from build123d import *

# Parameters (mm, degrees)
SKETCH_R        = 75
SKETCH_R_2      = 25
SKETCH_R_3      = 1.6
PAD_DEPTH       = 2.5
SKETCH001_W     = 23
SKETCH001_H     = 10
PAD001_DEPTH    = 15
SKETCH002_R     = 1.6
POCKET_DEPTH    = 130.001
SKETCH003_W     = 6
SKETCH003_H     = 3
POCKET001_DEPTH = 10


with BuildPart() as part:
    # Sketch → Pad (new body)
    with BuildSketch(Plane.XY):
        Circle(SKETCH_R)
        Circle(SKETCH_R_2, mode=Mode.SUBTRACT)
        with Locations((0, 30)):
            Circle(SKETCH_R_3, mode=Mode.SUBTRACT)
        with Locations((-25.980762, -15)):
            Circle(SKETCH_R_3, mode=Mode.SUBTRACT)
        with Locations((25.980762, -15)):
            Circle(SKETCH_R_3, mode=Mode.SUBTRACT)
    extrude(amount=PAD_DEPTH)

    # Sketch001 → Pad001 (new body)
    with BuildSketch(Plane.XY.offset(2.5)):
        with Locations((-31.5, 50)):
            Rectangle(SKETCH001_W, SKETCH001_H)
        with Locations((31.5, 50)):
            Rectangle(SKETCH001_W, SKETCH001_H)
        with Locations((-31.5, -50)):
            Rectangle(SKETCH001_W, SKETCH001_H)
        with Locations((31.5, -50)):
            Rectangle(SKETCH001_W, SKETCH001_H)
    extrude(amount=PAD001_DEPTH)

    # Sketch002 → Pocket (cut, through all)
    with BuildSketch(Plane.XZ.offset(55)):
        with Locations((31.5, 10.4)):
            Circle(SKETCH002_R)
        with Locations((-31.5, 10.4)):
            Circle(SKETCH002_R)
    extrude(amount=-POCKET_DEPTH, mode=Mode.SUBTRACT)

    # Sketch003 → Pocket001 (cut)
    with BuildSketch(Plane.XY.offset(17.5)):
        with Locations((31.5, -50)):
            Rectangle(SKETCH003_W, SKETCH003_H)
        with Locations((-31.5, -50)):
            Rectangle(SKETCH003_W, SKETCH003_H)
        with Locations((31.5, 50)):
            Rectangle(SKETCH003_W, SKETCH003_H)
        with Locations((-31.5, 50)):
            Rectangle(SKETCH003_W, SKETCH003_H)
    extrude(amount=-POCKET001_DEPTH, mode=Mode.SUBTRACT)


solid = part.part
Read the model definition and answer for the solid it produces. Units are mm, in the model's axes. A direction names the side the tool comes from. Give positions to 0.01 mm unless a question says otherwise; leave off trailing zeros. Write each loop counter-clockwise with the first axis right and the second up, starting at its lowest first coordinate (ties: lowest second). Pieces come first, ordered by that corner, then holes. Notation, with made-up numbers: (25, 26) - (29, 26) arc R11 cw to (29, 44) - close; hole circle Ø2 at (53.5, 72.25). An arc over 180 degrees is marked (long way). Use CSV: the item, a comma, the result in double quotes. Start each with the question number.
Item 1: Flat-ended cylindrical pins translate along their axes: P1, Ø0.9, axis at y = 50.5, z = 15, coming from the -X side; P2, Ø3, axis at x = -26, z = 14.5, coming from the +Y side; P3, Ø0.9, axis at x = 32, y = -49.5, coming from the +Z side; P4, Ø1.9, axis at x = -31.5, z = 10.4, coming from the +Y side. Find the tip coordinate at first contact, or state that the pin passes through.
Item 2: The mould has two halves that part along Z. Classify faces 1 (the cylindrical face through (-32.77, -53.27, 9.43)), 2 (the cylindrical face through (30.23, 46.73, 9.43)), 3 (the flat face through (-18, 18, 2.5)), 4 (the cylindrical face through (24.8, -13.92, 1.23)): pulls with the +Z half, pulls with the -Z half, needs draft (parallel to the pull), parting line crosses it, or undercut.
Item 3: The part is cut by section A-A, the plane y = 0. Give the vertices of the cut face in (x, z), and give its area (3 significant figures).
Item 4: The part is cut by section D-D, the plane y = -63. Give the vertices of the cut face in (x, z).
Item 5: The part is cut by section B-B, the plane x = -8.5. Give the vertices of the cut face in (y, z), and give its area (3 significant figures).
Item 6: For faces 5 (the flat face through (-32, -45, 8)), 6 (the flat face through (31, -48.5, 13)), 7 (the flat face through (43, 50, 10)), 8 (the flat face through (-32, -55, 8)), 9 (the flat face through (-43, 50, 10)), determine the directions among +Z, -Z, +X, -X, +Y, -Y from which every point of the face is accessible in a straight line to the end or side of a thin tool.
Item 7: Consider line 1 (X direction, y = 48, z = 16); line 2 (Y direction, x = 23.5, z = 10); line 3 (Z direction, x = -31.5, y = 45.8). Determine where each line is inside the solid, lowest interval first.
Item 8: The part is cut by section C-C, the plane x = 37. Give the vertices of the cut face in (y, z), and give its area (3 significant figures).
Taken from the geometry:
1,P1,"x = -43"
1,P2,"y = 55"
1,P3,"z = 7.5"
1,P4,"through"
2,face 1,"undercut"
2,face 2,"undercut"
2,face 3,"pulls with the +Z half"
2,face 4,"needs draft"
3,outline,"(-75, 0) - (-25, 0) - (-25, 2.5) - (-75, 2.5) - close; (25, 0) - (75, 0) - (75, 2.5) - (25, 2.5) - close"
3,area,"250 mm2"
4,outline,"(-40.69, 0) - (40.69, 0) - (40.69, 2.5) - (-40.69, 2.5) - close"
5,outline,"(-74.52, 0) - (-23.51, 0) - (-23.51, 2.5) - (-74.52, 2.5) - close; (23.51, 0) - (74.52, 0) - (74.52, 2.5) - (23.51, 2.5) - close"
5,area,"255 mm2"
6,face 5,"+Z, +X, -X"
6,face 6,"+Z"
6,face 7,"+Z, +X, +Y, -Y"
6,face 8,"+Z, +X, -X, -Y"
6,face 9,"+Z, -X, +Y, -Y"
7,line 1,"-43 to -20, 20 to 43"
7,line 2,"-55 to -45, 45 to 55"
7,line 3,"0 to 8.8, 12 to 17.5"
8,outline,"(-65.24, 0) - (65.24, 0) - (65.24, 2.5) - (55, 2.5) - (55, 17.5) - (45, 17.5) - (45, 2.5) - (-45, 2.5) - (-45, 17.5) - (-55, 17.5) - (-55, 2.5) - (-65.24, 2.5) - close"
8,area,"626 mm2"
